Check sheet for the modelled part. Datum: model origin and axes. Units: mm. A direction names the side the tool comes from. Round coordinates to 2 decimals unless told otherwise and drop trailing zeros. Order: outer loops, then holes, each group sorted by start corner. A loop starts at its lowest first (then second) coordinate and runs counter-clockwise, first axis right, second up.
```python
from build123d import *

# Parameters (mm, degrees)
SKETCH1_R           = 4.25
BOSS_EXTRUDE1_DEPTH = 3
CHAMFER1_SIZE       = 12
FILLET1_R           = 10
FILLET2_R           = 10


with BuildPart() as part:
    # Sketch1 → Boss-Extrude1 (new body)
    with BuildSketch(Plane.XY):
        Polygon((0, 30), (0, 0), (60, 0), (60, 30), (36, 30), (36, 10), (10, 10), (10, 30), align=None)
        with Locations((52, 18)):
            Circle(SKETCH1_R, mode=Mode.SUBTRACT)
    extrude(amount=BOSS_EXTRUDE1_DEPTH)

    # Chamfer1
    chamfer1_edges = [part.edges().sort_by_distance(p)[0] for p in [
        (60, 0, 1.5),
    ]]
    chamfer(chamfer1_edges, length=CHAMFER1_SIZE)

    # Fillet1
    fillet1_edges = [part.edges().sort_by_distance(p)[0] for p in [
        (60, 30, 1.5),
    ]]
    fillet(fillet1_edges, radius=FILLET1_R)

    # Fillet2
    fillet2_edges = [part.edges().sort_by_distance(p)[0] for p in [
        (60, 12, 1.5),
        (48, 0, 1.5),
    ]]
    fillet(fillet2_edges, radius=FILLET2_R)


solid = part.part
```
Item 1: Sectioned sample at D-D (x = 17). Record the cut outline in (y, z).
Answer:
outline: (0, 0) - (10, 0) - (10, 3) - (0, 3) - close
Item 2: Release check for a two-part mould opening along X. For faces 1 (the flat face through (30, 9, 3)), 2 (the flat face through (36, 20, 1)), 3 (the cylindrical face through (59.26, 12.37, 1.52)), 4 (the flat face through (10, 20, 1)) record: released by +X, released by -X, zero draft, split by the parting line, or undercut.
Answer:
face 1: zero draft
face 2: undercut
face 3: released by +X
face 4: undercut
Item 3: Go/stop test with flat-tipped pins: P1, Ø6, axis at x = 6.5, y = 9.5, coming from the -Z side; P2, Ø1.5, axis at x = 20, z = 1.5, coming from the +Y side. Record where each tip stops, or that it passes through.
Answer:
P1: stops at z = 0
P2: stops at y = 10
Item 4: Access from +Z, -Z, +X, -X, +Y, -Y to the whole of each face (thin tool, end or side, straight path). Record for faces 5 (the flat face through (43, 30, 1)), 6 (the flat face through (23, 10, 1)).
Answer:
face 5: +Z, -Z, +X, -X, +Y
face 6: +Z, -Z, +Y
Item 5: Scan lines: line 1 along Y through (x, z) = (52, 1.05); line 2 along X through (y, z) = (15.5, 2.9); line 3 along Y through (x, z) = (54, 1.7). Record each from-to range of solid material in increasing order.
Answer:
line 1: y = 4 to 13.75, 22.25 to 29.8
line 2: x = 0 to 10, 36 to 48.56, 55.44 to 59.98
line 3: y = 6 to 14.25, 21.75 to 29.17
Item 6: Sectioned sample at A-A (z = 1.95). Record the cut outline in (x, y).
Answer:
outline: (0, 0) - (43.86, 0) arc R10 ccw to (50.93, 2.93) - (57.07, 9.07) arc R10 ccw to (60, 16.14) - (60, 20) arc R10 ccw to (50, 30) - (36, 30) - (36, 10) - (10, 10) - (10, 30) - (0, 30) - close; hole circle Ø8.5 at (52, 18)
Item 7: Sectioned sample at B-B (y = 18). Record the cut outline in (x, z), and give its area (3 significant figures).
Answer:
outline: (0, 0) - (10, 0) - (10, 3) - (0, 3) - close; (36, 0) - (47.75, 0) - (47.75, 3) - (36, 3) - close; (56.25, 0) - (60, 0) - (60, 3) - (56.25, 3) - close
area: 76.5 mm2
Item 8: Sectioned sample at C-C (x = 52). Record the cut outline in (y, z), and give its area (3 significant figures).
Answer:
outline: (4, 0) - (13.75, 0) - (13.75, 3) - (4, 3) - close; (22.25, 0) - (29.8, 0) - (29.8, 3) - (22.25, 3) - close
area: 51.9 mm2
